```python
from build123d import *

# Parameters (mm, degrees)
F0_W      = 417
F0_H      = 63
F15_DEPTH = 6
F16_DEPTH = 3
F17_R     = 5


with BuildPart() as f15:
    # F0 (on Top) → F15 (new body)
    with BuildSketch(Plane.XY):
        with Locations((76.4282132271, 31.5)):
            Rectangle(F0_W, F0_H)
    extrude(amount=F15_DEPTH)

    # F1 (on Top) + F2 (on Top) + F3 (on Top) + F4 (on Top) + F5 (on Top) + F6 (on Top) + F7 (on Top) + F8 (on face) + F9 (on face) + F10 (on face) + F11 (on face) + F12 (on face) + F13 (on face) + F14 (on face) → F16 (cut)
    with BuildSketch(Plane.XY):
        Polygon((250.4282132271, 59), (225.9282132271, 34.5), (225.9282132271, 28.5), (250.4282132271, 4), (256.4282132271, 4), (280.9282132271, 28.5), (280.9282132271, 34.5), (256.4282132271, 59), align=None)
    with BuildSketch(Plane.XY):
        Polygon((191.4282132271, 59), (166.9282132271, 34.5), (166.9282132271, 28.5), (191.4282132271, 4), (197.4282132271, 4), (221.9282132271, 28.5), (221.9282132271, 34.5), (197.4282132271, 59), align=None)
    with BuildSketch(Plane.XY):
        Polygon((132.4282132271, 59), (107.9282132271, 34.5), (107.9282132271, 28.5), (132.4282132271, 4), (138.4282132271, 4), (162.9282132271, 28.5), (162.9282132271, 34.5), (138.4282132271, 59), align=None)
    with BuildSketch(Plane.XY):
        Polygon((73.4282150233, 59), (48.9282132271, 34.5000017962), (48.9282132271, 28.5000017962), (73.4282114309, 4), (79.4282114309, 4), (103.9282132271, 28.4999982038), (103.9282132271, 34.4999982038), (79.4282150233, 59), align=None)
    with BuildSketch(Plane.XY):
        Polygon((14.4282143313, 59), (-10.0717867729, 34.5000011042), (-10.0717867729, 28.5000011042), (14.4282121229, 4), (20.4282121229, 4), (44.9282132271, 28.4999988958), (44.9282132271, 34.4999988958), (20.4282143313, 59), align=None)
    with BuildSketch(Plane.XY):
        Polygon((-44.5717858043, 59), (-69.0717867729, 34.5000009686), (-69.0717867729, 28.5000009686), (-44.5717877415, 4), (-38.5717877415, 4), (-14.0717867729, 28.4999990314), (-14.0717867729, 34.4999990314), (-38.5717858043, 59), align=None)
    with BuildSketch(Plane.XY):
        Polygon((-103.5717843258, 59), (-128.0717867729, 34.5000024471), (-128.0717867729, 28.5000024471), (-103.57178922, 4), (-97.57178922, 4), (-73.0717867729, 28.4999975529), (-73.0717867729, 34.4999975529), (-97.5717843258, 59), align=None)
    with BuildSketch(Plane.XY):
        Polygon((245.2491989162, 9.1790143109), (231.1070632925, 23.3211499346), (227.5715293866, 19.7856160287), (241.7136650103, 5.6434804049), align=None)
    with BuildSketch(Plane.XY):
        Polygon((186.2366352396, 9.1915779875), (172.0944996159, 23.3337136112), (168.55896571, 19.7981797053), (182.7011013337, 5.6560440815), align=None)
    with BuildSketch(Plane.XY):
        Polygon((127.2366352396, 9.1915779875), (113.0944996159, 23.3337136112), (109.55896571, 19.7981797053), (123.7011013337, 5.6560440815), align=None)
    with BuildSketch(Plane.XY):
        Polygon((68.2493617452, 9.1788504451), (54.1072271583, 23.3209871057), (50.5716929931, 19.7854534589), (64.71382758, 5.6433167984), align=None)
    with BuildSketch(Plane.XY):
        Polygon((9.2493622909, 9.1788502988), (-4.8927726955, 23.3209865599), (-8.4283067607, 19.7854528133), (5.7138282256, 5.6433165522), align=None)
    with BuildSketch(Plane.XY):
        Polygon((-49.7506376022, 9.1788502702), (-63.8927726668, 23.320986453), (-67.4283067125, 19.7854526868), (-53.2861716479, 5.643316504), align=None)
    with BuildSketch(Plane.XY):
        Polygon((-108.7506387682, 9.1788505827), (-122.8927729793, 23.320987619), (-126.4283072384, 19.7854540662), (-112.2861730272, 5.6433170299), align=None)
    extrude(amount=F16_DEPTH, mode=Mode.SUBTRACT)

    # F17
    f17_edges = [f15.edges().sort_by_distance(p)[0] for p in [
        (284.928213, 0, 3),
        (284.928213, 63, 3),
        (-132.071787, 63, 3),
        (-132.071787, 0, 3),
    ]]
    fillet(f17_edges, radius=F17_R)


solid = f15.part
```
Design review of the part built by this model. Coordinates are the model's own, in mm. Coordinates: 2 decimals unless noted, no trailing zeros. Loops run counter-clockwise (first coordinate to the right, second up) from the corner with the lowest first, then second, coordinate; pieces in that order, holes last. Notation, with made-up numbers: (62, 84) -> (117, 84) arc R33 cw to (117, 115) -> close; hole circle Ø11 at (12.5, 1). An arc over 180 degrees is marked (long way). Answer as a JSON object with one key per item and string values.
Q1. Take a section at B-B on x = 60.5. Give the boundary of the cut face in (y, z).
Answer block:
{"outline": "(0, 0) -> (9.86, 0) -> (9.86, 3) -> (46.07, 3) -> (46.07, 0) -> (63, 0) -> (63, 6) -> (0, 6) -> close"}
Q2. Take a section at D-D on x = 218. Give the boundary of the cut face in (y, z), plus the area to 3 significant figures.
Answer block:
{"outline": "(0, 0) -> (24.57, 0) -> (24.57, 3) -> (38.43, 3) -> (38.43, 0) -> (63, 0) -> (63, 6) -> (0, 6) -> close", "area": "336 mm^2"}
Q3. To check wall thickness, follow L1, parallel to Y at x = 136, z = 0.95; L2, parallel to Z at x = -56, y = 38.5; L3, parallel to Y at x = 64.5, z = 2.5. State the ranges of each line that lie inside material, in increasing order.
Answer block:
{"L1": "y = 0 to 4, 59 to 63", "L2": "z = 3 to 6", "L3": "y = 0 to 5.86, 50.07 to 63"}
Q4. Take a section at C-C on z = 0.95. Give the number of separate pieces and of enclosed holes in the cut face, plus the area to 3 significant figures.
Answer block:
{"separate pieces": "1", "enclosed holes": "7", "area": "12,800 mm^2"}
